For this review, use the dimensioned drawing (mm, ordinates from the lowest corner) and the shaded views. A direction names the side the tool comes from. Coordinates: 2 decimals unless noted, no trailing zeros. Order: outer loops, then holes, each group sorted by start corner. A loop starts at its lowest first (then second) coordinate and runs counter-clockwise, first axis right, second up. Notation, with made-up numbers: (83.5, 43) -> (128.5, 43) arc R23 ccw to (128.5, 66) -> close; hole circle Ø5 at (64.25, -28). An arc over 180 degrees is marked (long way). Return JSON: item names as keys, results as strings. Group by question number.
Item 1: Machinability: for the marked faces 1, 2 and 3, which of the approach directions +Z, -Z, +X, -X, +Y, -Y give a long, thin tool a straight path to every point of the face, cutting with its end or side? Answer none if there is none.
Item 2: Take a section at A-A (z = 20). Write out the cut boundary in (x, y).
Item 3: Take a section at C-C (x = 23). Write out the cut boundary in (y, z), then the cut area to 3 significant figures.
Item 4: Take a section at B-B (y = 11.5). Write out the cut boundary in (x, z), then the cut area to 3 significant figures.
Item 5: Insertion check: pin 1 (7 mm diameter, centred on x = 17.5, y = 31.5, fed in from -Z); pin 2 (4 mm diameter, centred on x = 7.5, z = 20.5, fed in from +Y); pin 3 (5 mm diameter, centred on x = 8, y = 14, fed in from +Z). Each pin has a flat end and moves straight along its axis. Give the tip position at first contact, or say it passes through.
Item 6: Take a section at D-D (x = 4). Write out the cut boundary in (y, z).
Item 7: For line 1 along X through (y, z) = (9, 20); line 2 along Z through (x, y) = (19.5, 5); line 3 along Y through (x, z) = (18, 9.5), list the stretches that pass through material, from the lowest coordinate up.
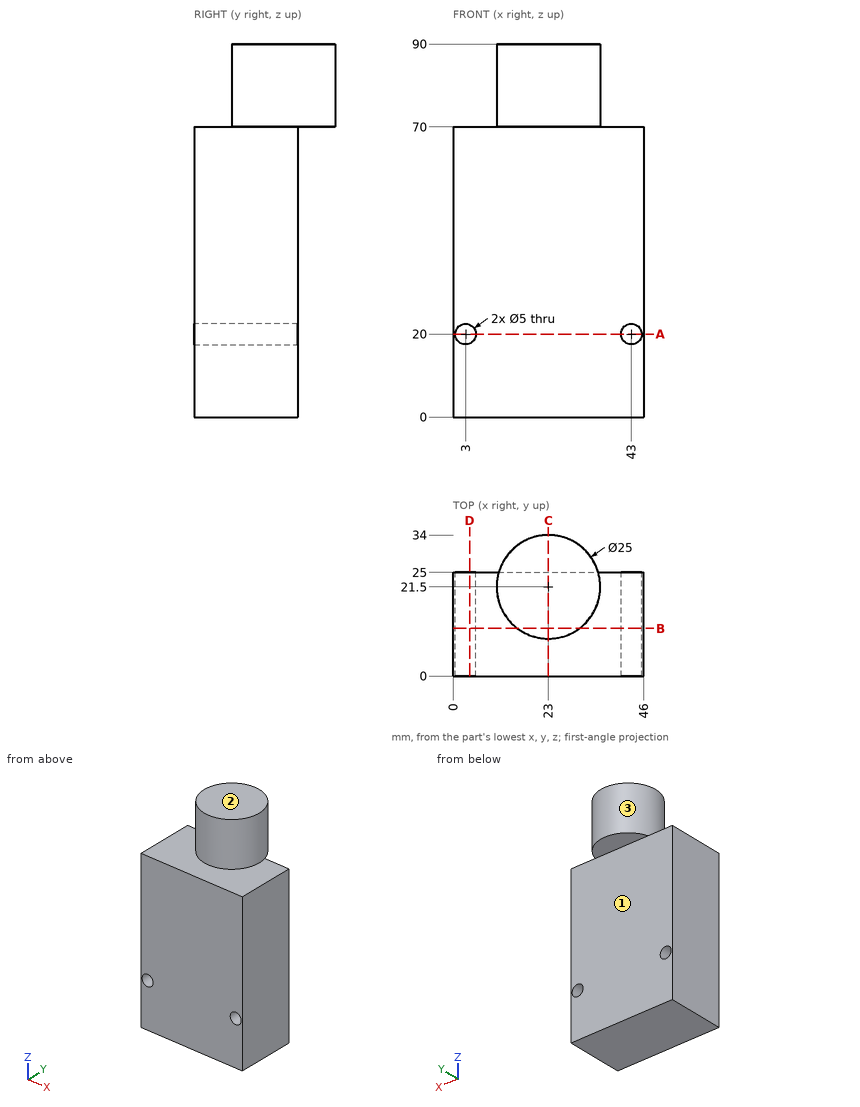
Findings below:
{
 "1": {"face 1": "-Z, +X, -X, +Y", "face 2": "+Z, +X, -X, +Y, -Y", "face 3": "+Z"},
 "2": {"outline": "(0, 0) -> (0.5, 0) -> (0.5, 25) -> (0, 25) -> close; (5.5, 0) -> (40.5, 0) -> (40.5, 25) -> (5.5, 25) -> close; (45.5, 0) -> (46, 0) -> (46, 25) -> (45.5, 25) -> close"},
 "3": {"outline": "(0, 0) -> (25, 0) -> (25, 70) -> (34, 70) -> (34, 90) -> (9, 90) -> (9, 70) -> (0, 70) -> close", "area": "2,250 mm2"},
 "4": {"outline": "(0, 0) -> (46, 0) -> (46, 70) -> (30.5, 70) -> (30.5, 90) -> (15.5, 90) -> (15.5, 70) -> (0, 70) -> close; hole circle Ø5 at (3, 20); hole circle Ø5 at (43, 20)", "area": "3,480 mm2"},
 "5": {"pin 1": "stops at z = 70", "pin 2": "stops at y = 25", "pin 3": "stops at z = 70"},
 "6": {"outline": "(0, 0) -> (25, 0) -> (25, 17.71) -> (0, 17.71) -> close; (0, 22.29) -> (25, 22.29) -> (25, 70) -> (0, 70) -> close"},
 "7": {"line 1": "x = 0 to 0.5, 5.5 to 40.5, 45.5 to 46", "line 2": "z = 0 to 70", "line 3": "y = 0 to 25"}
}
